For this review, take the finished solid that the model builds, in its own axes (mm). Face numbers are marked on the shaded views. A direction names the side the tool comes from. Give positions to 0.01 mm unless a question says otherwise; leave off trailing zeros. Order: outer loops, then holes, each group sorted by start corner. A loop starts at its lowest first (then second) coordinate and runs counter-clockwise, first axis right, second up. Notation, with made-up numbers: (38.25, -4.75) -> (65.25, -4.75) arc R18 cw to (65.25, 15.25) -> close; hole circle Ø11 at (3, -22). An arc over 180 degrees is marked (long way). One line per item, written item: value. Start each with the question number.
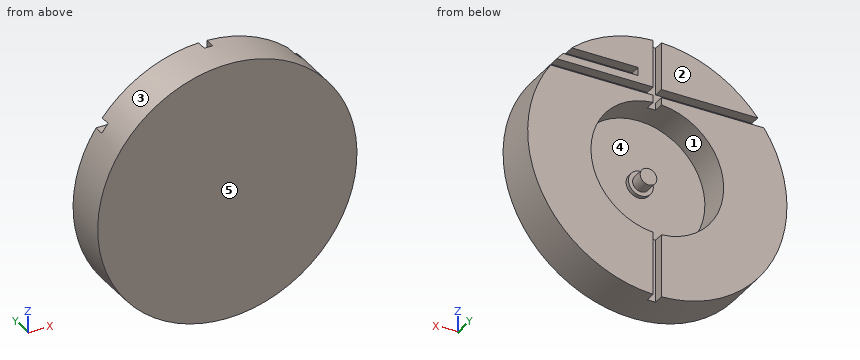
from build123d import *

# Parameters (mm, degrees)
SKETCH1_R           = 62.5
BOSS_EXTRUDE1_DEPTH = 21
SKETCH2_R           = 32
SKETCH2_R_2         = 6
CUT_EXTRUDE1_DEPTH  = 16
SKETCH3_R           = 6
SKETCH3_R_2         = 4
CUT_EXTRUDE2_DEPTH  = 14
SKETCH4_R           = 4
CUT_EXTRUDE3_DEPTH  = 7.5
CUT_EXTRUDE4_START  = -5
CUT_EXTRUDE4_DEPTH  = 5
CUT_EXTRUDE5_START  = -5
CUT_EXTRUDE5_DEPTH  = 5
CUT_EXTRUDE6_START  = -5
CUT_EXTRUDE6_DEPTH  = 5


with BuildPart() as part:
    # Sketch1 → Boss-Extrude1 (new body)
    with BuildSketch(Plane(origin=(0, 0, 0), x_dir=(1, 0, 0), z_dir=(0, 1, 0))):
        with Locations(Location((0, 0, 0), (0, 0, 90))):
            Circle(SKETCH1_R)
    extrude(amount=BOSS_EXTRUDE1_DEPTH)

    # Sketch2 → Cut-Extrude1 (cut)
    with BuildSketch(Plane(origin=(0, 21, 0), x_dir=(1, 0, 0), z_dir=(0, 1, 0))):
        with Locations(Location((0, 0, 0), (0, 0, 270))):
            Circle(SKETCH2_R)
        with Locations(Location((0, 0, 0), (0, 0, 270))):
            Circle(SKETCH2_R_2, mode=Mode.SUBTRACT)
    extrude(amount=-CUT_EXTRUDE1_DEPTH, mode=Mode.SUBTRACT)

    # Sketch3 → Cut-Extrude2 (cut)
    with BuildSketch(Plane(origin=(0, 21, 0), x_dir=(1, 0, 0), z_dir=(0, 1, 0))):
        with Locations(Location((0, 0, 0), (0, 0, 270))):
            Circle(SKETCH3_R)
        with Locations(Location((0, 0, 0), (0, 0, 270))):
            Circle(SKETCH3_R_2, mode=Mode.SUBTRACT)
    extrude(amount=-CUT_EXTRUDE2_DEPTH, mode=Mode.SUBTRACT)

    # Sketch4 → Cut-Extrude3 (cut)
    with BuildSketch(Plane(origin=(0, 21, 0), x_dir=(1, 0, 0), z_dir=(0, 1, 0))):
        with Locations(Location((0, 0, 0), (0, 0, 270))):
            Circle(SKETCH4_R)
    extrude(amount=-CUT_EXTRUDE3_DEPTH, mode=Mode.SUBTRACT)

    # Sketch5 → Cut-Extrude4 (cut)
    with BuildSketch(Plane(origin=(0, 21, 0), x_dir=(1, 0, 0), z_dir=(0, 1, 0)).offset(CUT_EXTRUDE4_START)):
        with BuildLine():
            Line((2, 62.467991804), (2, -62.467991804))
            ThreePointArc((2, -62.467991804), (0, -62.5), (-2, -62.467991804))
            Line((-2, -62.467991804), (-2, 62.467991804))
            ThreePointArc((-2, 62.467991804), (0, 62.5), (2, 62.467991804))
        make_face()
    extrude(amount=CUT_EXTRUDE4_DEPTH, mode=Mode.SUBTRACT)

    # Sketch6 → Cut-Extrude5 (cut)
    with BuildSketch(Plane(origin=(0, 21, 0), x_dir=(1, 0, 0), z_dir=(0, 1, 0)).offset(CUT_EXTRUDE5_START)):
        with BuildLine():
            Line((-48.435524153, -39.5), (48.435524153, -39.5))
            ThreePointArc((48.435524153, -39.5), (49.977438468, -37.530063205), (51.439284598, -35.5))
            Line((51.439284598, -35.5), (-51.439284598, -35.5))
            ThreePointArc((-51.439284598, -35.5), (-49.977438468, -37.530063205), (-48.435524153, -39.5))
        make_face()
    extrude(amount=CUT_EXTRUDE5_DEPTH, mode=Mode.SUBTRACT)

    # Sketch9 → Cut-Extrude6 (cut)
    with BuildSketch(Plane(origin=(0, 21, 0), x_dir=(1, 0, 0), z_dir=(0, 1, 0)).offset(CUT_EXTRUDE6_START)):
        with BuildLine():
            Line((41.19769411, -43), (45.356917885, -43))
            ThreePointArc((45.356917885, -43), (43.323494947, -45.048027544), (41.19769411, -47))
            Line((41.19769411, -47), (9.19769411, -47))
            Line((9.19769411, -47), (9.19769411, -43))
            Line((9.19769411, -43), (41.19769411, -43))
        make_face()
    extrude(amount=CUT_EXTRUDE6_DEPTH, mode=Mode.SUBTRACT)


solid = part.part
Q1. Take a section at B-B (x = 0). State the section outline as (y, z) points.
Q2. For line 1 along X through (y, z) = (11.25, 0); line 2 along X through (y, z) = (14.5, 0); line 3 along Y through (x, z) = (-13, -29), list the stretches that pass through material, from the lowest coordinate up.
Q3. Mouldability with a two-part tool opening along Z and no side actions: class the marked faces 1, 2 and 3 as pulls with the +Z half, pulls with the -Z half, needs draft (parallel to the pull), parting line crosses it, or undercut.
Q4. For pin 1 Ø1.5 at (y, z) = (18.5, -47.5) entering from +X; pin 2 Ø4 at (y, z) = (18.5, 12.5) entering from +X; pin 3 Ø4 at (y, z) = (14.5, 46) entering from +X, all flat-tipped, find the tip position at first contact; note any pin that passes through.
Q5. For the marked faces 4 and 5, list the 3-axis set-ups (+Z, -Z, +X, -X, +Y, -Y) from which the entire face can be reached by the end or side of a thin tool; tool diameter is ignored.
Q6. Take a section at A-A (y = 9). State the section outline as (x, z) points.
Q7. Take a section at D-D (z = 23). State the section outline as (x, y) points, and give its area (3 significant figures).
Q8. Take a section at C-C (z = 0). State the section outline as (x, y) points, and give its area (3 significant figures).
Answers below:
1. outline: (0, -62.5) -> (16, -62.5) -> (16, -32) -> (5, -32) -> (5, -6) -> (7, -6) -> (7, -4) -> (13.5, -4) -> (13.5, 4) -> (7, 4) -> (7, 6) -> (5, 6) -> (5, 32) -> (16, 32) -> (16, 62.5) -> (0, 62.5) -> close
2. line 1: x = -62.5 to -32, -4 to 4, 32 to 62.5
2. line 2: x = -62.5 to -32, 32 to 62.5
2. line 3: y = 0 to 5
3. face 1: undercut
3. face 2: needs draft
3. face 3: parting line crosses it
4. pin 1: stops at x = 41.48
4. pin 2: stops at x = 61.61
4. pin 3: stops at x = 44.39
5. face 4: +Y
5. face 5: +Z, -Z, +X, -X, -Y
6. outline: circle Ø125 at (0, 0); circle Ø8 at (0, 0); hole circle Ø64 at (0, 0)
7. outline: (-58.11, 0) -> (58.11, 0) -> (58.11, 21) -> (22.25, 21) -> (22.25, 5) -> (-22.25, 5) -> (-22.25, 21) -> (-58.11, 21) -> close
7. area: 1,730 mm²
8. outline: (-62.5, 0) -> (62.5, 0) -> (62.5, 21) -> (32, 21) -> (32, 5) -> (6, 5) -> (6, 7) -> (4, 7) -> (4, 13.5) -> (-4, 13.5) -> (-4, 7) -> (-6, 7) -> (-6, 5) -> (-32, 5) -> (-32, 21) -> (-62.5, 21) -> close
8. area: 1,680 mm²
